Check sheet for the modelled part. Datum: model origin and axes. Units: mm. Coordinates: 2 decimals unless noted, no trailing zeros. Write each loop counter-clockwise with the first axis right and the second up, starting at its lowest first coordinate (ties: lowest second). Pieces come first, ordered by that corner, then holes. Notation, with made-up numbers: M -33.5,77 L -18.5,77 A12 ccw -18.5,84 Z; hole C -40,11.25 d6. An arc over 180 degrees is marked long. Answer as CSV lines item,"result". Start each with the question number.
1) Section check A-A (x = 0). Record the cut outline in (y, z).
2) Material ranges on L1, parallel to Z at x = 4.5, y = 5; L2, parallel to Y at x = 0.25, z = 76; L3, parallel to Y at x = -3.5, z = 128, recorded low to high. Write a range as [from, to].
3) Go/stop test with flat-tipped pins: pin 1 Ø1.5 at (x, z) = (-1, 130.5) entering from -Y; pin 2 Ø1 at (y, z) = (-1.5, 155.5) entering from +X; pin 3 Ø4 at (x, z) = (6, 122.5) entering from +Y. Record where each tip stops, or that it passes through.
4) Section check B-B (z = 82). Record the cut outline in (x, y), and give its area (3 significant figures).
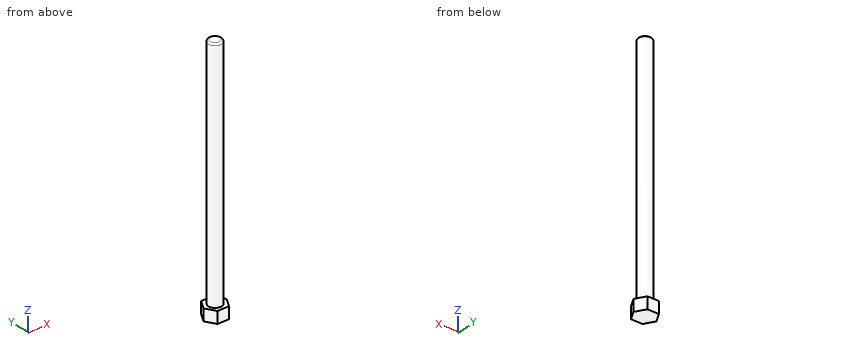
from build123d import *

# Parameters (mm, degrees)
F0_R     = 4.74599
F1_DEPTH = 177.8
F3_DEPTH = 8.334375
F4_R     = 1.27


# Not quite as in the source:
# - a length typed as a fraction of an inch, garbled in the dataset ("3 / 203.2 mm" for 3/8 in), is restored


with BuildPart() as f1:
    # F0 (on Top) → F1 (new body)
    with BuildSketch(Plane.XY):
        Circle(F0_R)
    extrude(amount=F1_DEPTH)

    # F2 (on Top) → F3 (join)
    with BuildSketch(Plane.XY):
        Polygon((-4.1244459855, -7.14375), (4.1244459855, -7.14375), (8.248891971, 0), (4.1244459855, 7.14375), (-4.1244459855, 7.14375), (-8.248891971, 0), align=None)
    extrude(amount=F3_DEPTH)

    # F4
    f4_edges = [f1.edges().sort_by_distance(p)[0] for p in [
        (-4.74599, 0, 177.8),
    ]]
    fillet(f4_edges, radius=F4_R)


solid = f1.part
Results found:
1,outline,"M -7.14,0 L 7.14,0 L 7.14,8.33 L 4.75,8.33 L 4.75,176.53 A1.27 ccw 3.48,177.8 L -3.48,177.8 A1.27 ccw -4.75,176.53 L -4.75,8.33 L -7.14,8.33 Z"
2,L1,"z = [0, 8.33]"
2,L2,"y = [-4.74, 4.74]"
2,L3,"y = [-3.21, 3.21]"
3,pin 1,"stops at y = -4.74"
3,pin 2,"stops at x = 4.64"
3,pin 3,"stops at y = 2.55"
4,outline,"C 0,0 d9.49"
4,area,"70.8 mm2"
